Input: dimensioned drawing with shaded views. Units: mm. Origin: part minimum x, y, z. A direction names the side the tool comes from. Round coordinates to 2 decimals unless told otherwise and drop trailing zeros. Loops run counter-clockwise (first coordinate to the right, second up) from the corner with the lowest first, then second, coordinate; pieces in that order, holes last.
Item 1: Section query A-A on y = 10.5. Return loops of the section in (x, z).
Item 2: Section query B-B on z = 4. Give the number of separate pieces and of enclosed holes in the cut face, then the cut area to 3 significant figures.
Item 3: Section query D-D on y = 113.5. Return loops of the section in (x, z).
Item 4: Pull-direction query (X, two-part tool) for the marked faces 1 and 2; classes: released by +X, released by -X, zero draft, split by the parting line, or undercut.
Item 5: Access query for the marked faces 3, 4, 5 and 6. Directions: +Z, -Z, +X, -X, +Y, -Y. A direction counts if a zero-diameter tool reaches every point of the face in a straight line with its end or side. Return the directions, or none.
Item 6: Section query C-C on y = 81. Return loops of the section in (x, z), then the cut area to 3 significant figures.
Item 7: First-contact query: P1, Ø7.5, axis at x = 45, z = 7, coming from the +Y side; P2, Ø1, axis at x = 54, z = 6, coming from the -Y side; P3, Ø4.5, axis at x = 145, z = 10, coming from the -Y side; P4, Ø5, axis at y = 116.5, z = 5.5, coming from the +X side. Flat tips, straight axial feed; report the tip coordinate or a pass-through.
Item 8: Ray query, L1, parallel to X at y = 11, z = 8; L2, parallel to Y at x = 69, z = 4. Return the intervals inside material, ascending.
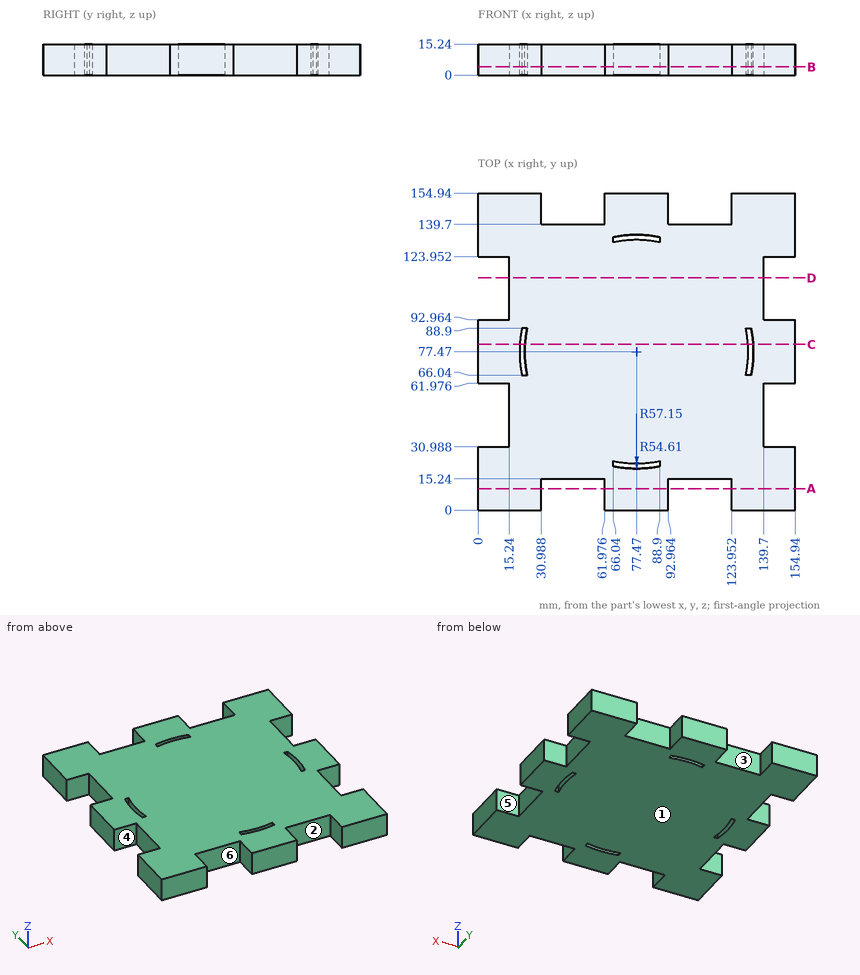
Data:
1. outline: (0, 0) - (30.99, 0) - (30.99, 15.24) - (0, 15.24) - close; (61.98, 0) - (92.96, 0) - (92.96, 15.24) - (61.98, 15.24) - close; (123.95, 0) - (154.94, 0) - (154.94, 15.24) - (123.95, 15.24) - close
2. separate pieces: 1
2. enclosed holes: 4
2. area: 20,000 mm2
3. outline: (15.24, 0) - (139.7, 0) - (139.7, 15.24) - (15.24, 15.24) - close
4. face 1: zero draft
4. face 2: undercut
5. face 3: +Z, -Z, +Y
5. face 4: +Z, -Z, -X
5. face 5: +Z, -Z, +X
5. face 6: +Z, -Z, -Y
6. outline: (0, 0) - (20.43, 0) - (20.43, 15.24) - (0, 15.24) - close; (22.97, 0) - (131.97, 0) - (131.97, 15.24) - (22.97, 15.24) - close; (134.51, 0) - (154.94, 0) - (154.94, 15.24) - (134.51, 15.24) - close
6. area: 2,280 mm2
7. P1: stops at y = 139.7
7. P2: stops at y = 15.24
7. P3: stops at y = 0
7. P4: stops at x = 139.7
8. L1: x = 0 to 30.99, 61.98 to 92.96, 123.95 to 154.94
8. L2: y = 0 to 20.95, 23.52 to 131.42, 133.99 to 154.94
